Autodesk Inventor part; units mm, degrees
ref_plane "YZ Plane" through (0, 0, 0) normal (1, 0, 0) x (0, 1, 0)
ref_plane "XZ Plane" through (0, 0, 0) normal (0, 1, 0) x (-1, 0, 0)
ref_plane "XY Plane" through (0, 0, 0) normal (0, 0, 1) x (1, 0, 0)
sketch "スケッチ1" plane through (0, 0, 0) normal (1, 0, 0) x (0, 1, 0)
  line L0 (0, 7.6073) -> (0, 0)
  line L1 (0, 0) -> (2.3241, 0)
  line L2 (2.3241, 0) -> (2.3241, 2.8448)
  line L3 (2.3241, 2.8448) -> (1.4, 2.8448)
  line L4 (1.4, 2.8448) -> (1.4, 7.6073)
  line L5 (1.4, 7.6073) -> (0, 7.6073)
  dimension "d1" = 1.4
  dimension "d2" = 2.8448
  dimension "d3" = 2.3241
  dimension "d10" = 4.7625
revolve "回転1" add sketch "スケッチ1" angle 360 about axis through (0, 0, 7.6073) along (0, 0, -1)
sketch "スケッチ2" plane through (0, 0, 0) normal (0, 0, -1) x (-1, 0, 0)
  line L0 (0, 1.3799) -> (1.195, 0.6899)
  line L1 (1.195, 0.6899) -> (1.195, -0.6899)
  line L2 (1.195, -0.6899) -> (0, -1.3799)
  line L3 (0, -1.3799) -> (-1.195, -0.6899)
  line L4 (-1.195, -0.6899) -> (-1.195, 0.6899)
  line L5 (-1.195, 0.6899) -> (0, 1.3799)
  circle A0 centre (0, 0) radius 2.3241
  line L6 (0, 2.3241) -> (0, -2.3241) construction
  point P0 (0, 0)
  dimension "d7" = 2.39
extrude "押し出し1" cut sketch "スケッチ2" against normal blind 1.4 contours L0 L1 L2 L3 L4 L5
thread "ねじ1"
properties part number "No4_40-3-16" material "ステンレス鋼 AISI 304"
For this review, take the finished solid that the model builds, in its own axes (mm). A direction names the side the tool comes from. Give positions to 0.01 mm unless a question says otherwise; leave off trailing zeros. Loops run counter-clockwise (first coordinate to the right, second up) from the corner with the lowest first, then second, coordinate; pieces in that order, holes last. Notation, with made-up numbers: (-38, 22.5) - (6, 22.5) arc R34 cw to (6, 52.5) - close; hole circle Ø4 at (18, 36). An arc over 180 degrees is marked (long way). Write each question's results on one line, items separated by ' | '.
(1) Draft analysis for pull direction X (two halves, no side actions). For faces 1 (the flat face through (1.195, 0, 1)), 2 (the flat face through (0, 0, 7.607)), 3 (the cylindrical face through (2.27, -0.5, 1.44)), state which applies: +X half, -X half, draft (parallel to the pull), parting line (faces both ways), or undercut.
Conclusion:
face 1: undercut | face 2: draft | face 3: parting line
(2) For faces 4 (the flat face through (0.59, -1.04, 0.69)), 5 (the flat face through (1, -1, 0)), 6 (the cylindrical face through (-0.06, -1.4, 5.26)), list the 3-axis set-ups (+Z, -Z, +X, -X, +Y, -Y) from which the entire face can be reached by the end or side of a thin tool; tool diameter is ignored.
Conclusion:
face 4: -Z | face 5: -Z, +X, -X, +Y, -Y | face 6: +Z
(3) Take a section at B-B (x = 0.35). Give the boundary of the cut face in (y, z).
Conclusion:
outline: (-2.3, 0) - (-1.18, 0) - (-1.18, 1.4) - (1.18, 1.4) - (1.18, 0) - (2.3, 0) - (2.3, 2.84) - (1.36, 2.84) - (1.36, 7.61) - (-1.36, 7.61) - (-1.36, 2.84) - (-2.3, 2.84) - close
(4) Take a section at A-A (y = 0). Give the boundary of the cut face in (x, z) (3 decimals).
Conclusion:
outline: (-2.324, 0) - (-1.195, 0) - (-1.195, 1.4) - (1.195, 1.4) - (1.195, 0) - (2.324, 0) - (2.324, 2.845) - (1.4, 2.845) - (1.4, 7.607) - (-1.4, 7.607) - (-1.4, 2.845) - (-2.324, 2.845) - close
(5) Take a section at C-C (z = 6.5). Give the boundary of the cut face in (x, y).
Conclusion:
outline: circle Ø2.8 at (0, 0)
(6) For pin 1 Ø1 at (x, z) = (0, 6) entering from -Y, flat-tipped, find the tip position at first contact; note if it passes through.
Conclusion:
pin 1: y = -1.4
(7) Take a section at D-D (y = 1.9). Give the boundary of the cut face in (x, z), then the cut area to 3 significant figures.
Conclusion:
outline: (-1.34, 0) - (1.34, 0) - (1.34, 2.84) - (-1.34, 2.84) - close | area: 7.62 mm^2
(8) For line 1 along Z through (x, y) = (0.8, -1.9); line 2 along Z through (x, y) = (0.6, -0.25); line 3 along Y through (x, z) = (-0.55, 0.5), list the stretches that pass through material, from the lowest coordinate up.
Conclusion:
line 1: 0 to 2.84 | line 2: 1.4 to 7.61 | line 3: -2.26 to -1.06, 1.06 to 2.26
